Can you work these out from the model? Positions are in its coordinate system, mm. A direction names the side the tool comes from. Round coordinates to 2 decimals unless told otherwise and drop trailing zeros. Loops run counter-clockwise (first coordinate to the right, second up) from the corner with the lowest first, then second, coordinate; pieces in that order, holes last.
```python
from build123d import *

# Parameters (mm, degrees)
SKETCH_R      = 2.55
PAD_DEPTH     = 6
SKETCH001_R   = 10
SKETCH001_R_2 = 2.55
PAD001_DEPTH  = 6
CHAMFER_SIZE  = 1
SKETCH002_R   = 2
POCKET_DEPTH  = 31.828851


with BuildPart() as part:
    # Sketch → Pad (new body)
    with BuildSketch(Plane.XY):
        with BuildLine():
            ThreePointArc((26.46873, -5.817459), (31, 0), (26.46873, 5.817459))
            Line((26.46873, 5.817459), (0, 12.5))
            Line((0, 12.5), (-26.46873, 5.817459))
            ThreePointArc((-26.46873, 5.817459), (-31, 0), (-26.46873, -5.817459))
            Line((-26.46873, -5.817459), (0, -12.5))
            Line((0, -12.5), (26.46873, -5.817459))
        make_face()
        Circle(SKETCH_R, mode=Mode.SUBTRACT)
        with Locations((-25, 0)):
            Circle(SKETCH_R, mode=Mode.SUBTRACT)
        with Locations((25, 0)):
            Circle(SKETCH_R, mode=Mode.SUBTRACT)
    extrude(amount=PAD_DEPTH)

    # Sketch001 (on Face11 of Pad) → Pad001 (join)
    with BuildSketch(Plane.XY.offset(6)):
        Circle(SKETCH001_R)
        Circle(SKETCH001_R_2, mode=Mode.SUBTRACT)
    extrude(amount=PAD001_DEPTH)

    # Chamfer
    chamfer_edges = [part.edges().sort_by_distance(p)[0] for p in [
        (-2.55, 0, 12),
    ]]
    chamfer(chamfer_edges, length=CHAMFER_SIZE)

    # Sketch002 (on Face8 of Chamfer) → Pocket (cut, through all)
    with BuildSketch(Plane(origin=(2.966762, 11.750984, 0), x_dir=(-0.969577, 0.244788, 0), z_dir=(0.244788, 0.969577, 0))):
        with Locations((0, 8.534735)):
            Circle(SKETCH002_R)
    extrude(amount=-POCKET_DEPTH, mode=Mode.SUBTRACT)


solid = part.part
```
(1) Suppose I cut it at D-D (x = 6). Write out the boundary of the cut face in (y, z).
(2) Which directions (+Z, -Z, +X, -X, +Y, -Y) give clear straight access to the entire face, cutting with the end or side of a thin tool? Please do faces 1 (the cylindrical face through (-1.302, 9.915, 8.958)), 2 (the flat face through (13.049, -9.206, 2.958)).
(3) For pin 1 (1.5 mm diameter, centred on x = 25, z = 1.5, fed in from -Y); pin 2 (4 mm diameter, centred on x = -24, z = 3.5, fed in from +Y); pin 3 (6.5 mm diameter, centred on x = 0, y = 0, fed in from +Z), each with a flat end and sliding along its axis, tell me the tip position at first contact or that it passes through.
(4) Suppose I cut it at C-C (z = 7.75). Write out the boundary of the cut face in (x, y), then the cut area to 3 significant figures.
(5) Suppose I cut it at A-A (y = 0). Write out the boundary of the cut face in (x, z).
(6) Suppose I cut it at B-B (x = 25). Write out the boundary of the cut face in (y, z).
(7) If I drill on line 1 (Y direction, x = 0, z = 3.25); line 2 (X direction, y = 1, z = 3.5); line 3 (Z direction, x = -12, y = 8), over which ranges is the centre line in solid material (lowest first)?
(8) We'd pull the mould along Y, two halves only. Please class faces 3 (the flat face through (-13.049, 9.206, 2.958)), 4 (the cylindrical face through (31, 0, 3)), 5 (the cylindrical face through (-3.195, -5.108, 7.769)): released by +Y, released by -Y, zero draft, split by the parting line, or undercut.
Check result:
1. outline: (-10.99, 0) - (10.99, 0) - (10.99, 6) - (8, 6) - (8, 12) - (-8, 12) - (-8, 6) - (-10.99, 6) - close
2. face 1: +Z
2. face 2: +Z, -Z, +X, -Y
3. pin 1: stops at y = -6.38
3. pin 2: stops at y = 6.95
3. pin 3: stops at z = 11.7
4. outline: (-4.19, -9.08) - (-2.22, -1.26) arc R2.55 cw to (-1.35, 2.16) - (0.62, 9.98) arc R10 ccw to start; (-0.62, -9.98) arc R10 ccw to (4.19, 9.08) - (2.22, 1.26) arc R2.55 cw to (1.35, -2.16) - close
4. area: 238 mm2
5. outline: (-31, 0) - (-27.55, 0) - (-27.55, 6) - (-31, 6) - close; (-22.45, 0) - (-2.55, 0) - (-2.55, 11) - (-3.55, 12) - (-10, 12) - (-10, 6) - (-22.45, 6) - close; (2.55, 0) - (22.45, 0) - (22.45, 6) - (10, 6) - (10, 12) - (3.55, 12) - (2.55, 11) - close; (27.55, 0) - (31, 0) - (31, 6) - (27.55, 6) - close
6. outline: (-6.19, 0) - (-2.55, 0) - (-2.55, 6) - (-6.19, 6) - close; (2.55, 0) - (6.19, 0) - (6.19, 6) - (2.55, 6) - close
7. line 1: y = -12.5 to -2.55, 2.55 to 12.5
7. line 2: x = -30.92 to -27.35, -22.65 to -2.35, 2.35 to 22.65, 27.35 to 30.92
7. line 3: z = 0 to 6
8. face 3: released by +Y
8. face 4: split by the parting line
8. face 5: undercut
